Read the model definition and answer for the solid it produces. Units are mm, in the model's axes. Face numbers are marked on the shaded views. A direction names the side the tool comes from. Coordinates: 2 decimals unless noted, no trailing zeros. Order: outer loops, then holes, each group sorted by start corner. A loop starts at its lowest first (then second) coordinate and runs counter-clockwise, first axis right, second up. Notation, with made-up numbers: M 72,-35 L 82,-35 A34 ccw 82,2 Z; hole C 64.25,-6 d1. An arc over 180 degrees is marked long. Write each question's results on one line, items separated by ' | '.
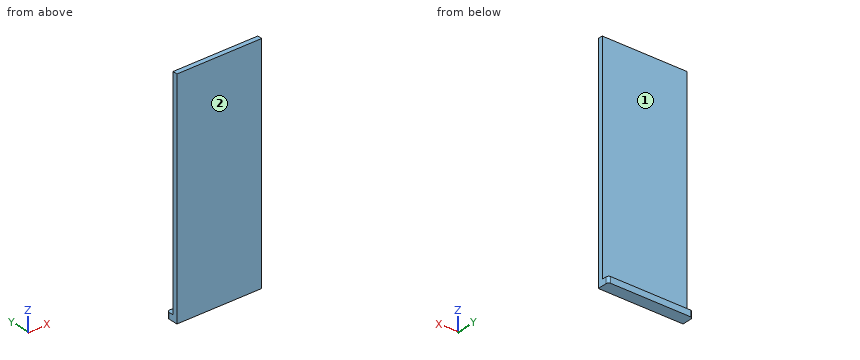
```python
from build123d import *

# Parameters (mm, degrees)
SLIDING_DOOR_SKETCH_W     = 88.9
SLIDING_DOOR_SKETCH_H     = 5.08
SLIDING_DOOR_HOLDER_DEPTH = 6.35
SKETCH1_5_W               = 88.9
SKETCH1_5_H               = 5.08
SLIDING_DOOR_DEPTH        = 234.95


with BuildPart() as part:
    # Sliding Door Sketch → Sliding Door Holder (new body)
    with BuildSketch(Plane.XY):
        with Locations((-0.46175508, 2.667)):
            Rectangle(SLIDING_DOOR_SKETCH_W, SLIDING_DOOR_SKETCH_H)
        with BuildLine():
            Line((-44.91175508, 10.287), (-44.91175508, 5.207))
            Line((-44.91175508, 5.207), (43.98824492, 5.207))
            Line((43.98824492, 5.207), (43.98824492, 10.287))
            ThreePointArc((43.98824492, 10.287), (43.244296144, 12.083051224), (41.44824492, 12.827))
            Line((41.44824492, 12.827), (-42.37175508, 12.827))
            ThreePointArc((-42.37175508, 12.827), (-44.167806304, 12.083051224), (-44.91175508, 10.287))
        make_face()
    extrude(amount=SLIDING_DOOR_HOLDER_DEPTH)

    # Sketch1_5 → Sliding Door (add)
    with BuildSketch(Plane.XY):
        with Locations((-0.46175508, 2.667)):
            Rectangle(SKETCH1_5_W, SKETCH1_5_H)
    extrude(amount=SLIDING_DOOR_DEPTH)


solid = part.part
```
(1) For the marked faces 1 and 2, determine the directions among +Z, -Z, +X, -X, +Y, -Y from which every point of the face is accessible in a straight line to the end or side of a thin tool.
Conclusion:
face 1: +Z, +X, -X, +Y | face 2: +Z, -Z, +X, -X, -Y
(2) The part is cut by section C-C, the plane y = 7.5. Write down the section's boundary in (x, z).
Conclusion:
outline: M -44.91,0 L 43.99,0 L 43.99,6.35 L -44.91,6.35 Z
(3) The part is cut by section A-A, the plane x = 31.5. Write down the section's boundary in (y, z), then the cut area to 3 significant figures.
Conclusion:
outline: M 0.13,0 L 12.83,0 L 12.83,6.35 L 5.21,6.35 L 5.21,234.95 L 0.13,234.95 Z | area: 1,240 mm²
(4) Given pin 1 (1.5 mm diameter, centred on x = -16, z = 174.5, fed in from +Y); pin 2 (3 mm diameter, centred on x = -33, y = 9, fed in from +Z), each flat-ended and moving along its own axis, determine where each tip first touches the part or whether it passes through.
Conclusion:
pin 1: y = 5.21 | pin 2: z = 6.35
(5) The part is cut by section B-B, the plane z = 196. Write down the section's boundary in (x, y), then the cut area to 3 significant figures.
Conclusion:
outline: M -44.91,0.13 L 43.99,0.13 L 43.99,5.21 L -44.91,5.21 Z | area: 452 mm²
(6) Straight lines are drawn through the part: line 1 (Y direction, x = -3.5, z = 66); line 2 (Z direction, x = 23.5, y = 6.5). For each, find the intervals that lie inside material, in ascending order.
Conclusion:
line 1: 0.13 to 5.21 | line 2: 0 to 6.35
